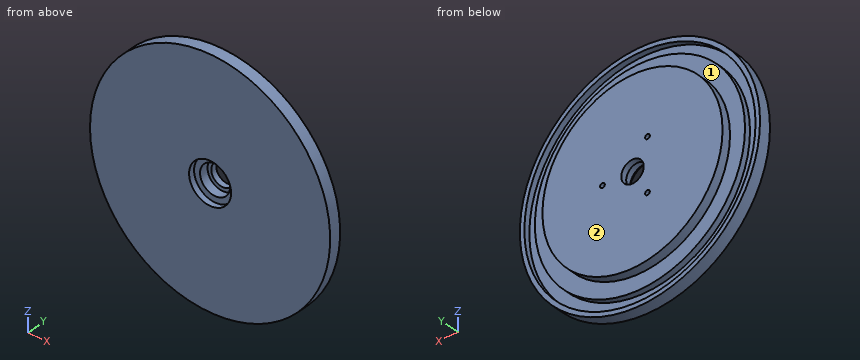
Autodesk Inventor part; units mm, degrees
ref_plane "YZ Plane" through (0, 0, 0) normal (1, 0, 0) x (0, 1, 0)
ref_plane "XZ Plane" through (0, 0, 0) normal (0, 1, 0) x (-1, 0, 0)
ref_plane "XY Plane" through (0, 0, 0) normal (0, 0, 1) x (1, 0, 0)
sketch "Sketch1" plane through (0, 0, 0) normal (0, 0, 1) x (1, 0, 0)
  line L0 (0, 0) -> (0, 5) construction
  line L1 (-40, 4) -> (-40, 0)
  line L2 (-40, 0) -> (-4.5, 0)
  line L3 (-38.5, 4) -> (-38.5, 2)
  line L4 (-38.5, 2) -> (-35, 2)
  line L5 (-35, 2) -> (-35, 4)
  line L6 (-30, 4) -> (-35, 4)
  line L7 (-38.5, 4) -> (-40, 4)
  line L8 (-3.75, 5) -> (-5, 5)
  line L9 (-5, 5) -> (-5, 2)
  line L10 (-3.5, 2.9949) -> (3.5, 2.9949)
  line L11 (3.5, 2.9949) -> (3.5, 2.0051)
  line L12 (3.5, 2.0051) -> (-3.5, 2.0051)
  line L13 (-3.5, 2.0051) -> (-3.5, 2.9949)
  line L14 (-3.5, 2.9949) -> (3.5, 2.0051) construction
  line L15 (3.5, 2.9949) -> (-3.5, 2.0051) construction
  line L16 (-30, 4) -> (-30, 7)
  line L17 (-30, 7) -> (-3.75, 7)
  line L18 (-3.75, 7) -> (-3.75, 5)
  line L19 (-5, 2) -> (-7, 2)
  line L20 (-7, 2) -> (-7, 0)
  point P0 (0, 2.5)
  dimension "d0" = 4
  dimension "d3" = 80
  dimension "d6" = 3.5
  dimension "d7" = 2
  dimension "d15" = 70
  dimension "d16" = 7
  dimension "d17" = 1.5
  dimension "d18" = 3
  dimension "d33" = 3
  dimension "d34" = 60
  dimension "d35" = 7.5
  dimension "d40" = 14
  dimension "d41" = 2
revolve "Revolution1" add sketch "Sketch1" angle 360 about axis through (0, 0, 0) along (0, 1, 0) contours L7 L3 L4 L5 L6 L16 L17 L18 L8 L9 L19 L20 L2 L1
sketch "Sketch3" plane through (0, 7, 0) normal (0, 1, 0) x (1, 0, 0)
  circle A0 centre (0, 0) radius 3.75
  point P0 (10, 0)
  dimension "d36" = 10
hole "Hole1" at (10, 7, 0) direction (0, -1, 0) diameter 1.567 depth 5 tip angle 118
pattern_circular "Circular Pattern2" count 3 over 360 about axis through (0, 5.5, 0) along (0, 1, 0) of "Hole1"
properties part number "007" material "Stainless Steel, 440C"
The listing builds one solid part. Answer for the finished solid, in the listing's coordinates (mm). Face numbers are marked on the shaded views. A direction names the side the tool comes from. Give positions to 0.01 mm unless a question says otherwise; leave off trailing zeros. Write each loop counter-clockwise with the first axis right and the second up, starting at its lowest first coordinate (ties: lowest second). Pieces come first, ordered by that corner, then holes.
Item 1: Section B-B, the plane z = -33.5 is taken. Write down the section's boundary in (x, y), plus the area to 3 significant figures.
Item 2: Section C-C, the plane x = 13 is taken. Write down the section's boundary in (y, z), plus the area to 3 significant figures.
Item 3: Section A-A, the plane x = 0 is taken. Write down the section's boundary in (y, z).
Item 4: Section D-D, the plane z = 11 is taken. Write down the section's boundary in (x, y).
Item 5: A flat-ended cylindrical pin translates along its axis: P1, Ø1.4, axis at x = -5, z = 8.66, coming from the +Y side. Find the tip coordinate at first contact, or state that the pin passes through.
Item 6: Find the intervals of material crossed by line 1 along Z through (x, y) = (0, 2.6); line 2 along Z through (x, y) = (-11.5, 3.5); line 3 along Z through (x, y) = (3, 2.5), in increasing order.
Item 7: Which of the six approach directions +Z, -Z, +X, -X, +Y, -Y give full straight-line access (tool end or side, diameter ignored) to the marked faces 1 and 2?
Completed:
1. outline: (-21.86, 0) - (21.86, 0) - (21.86, 4) - (18.97, 4) - (18.97, 2) - (10.14, 2) - (10.14, 4) - (-10.14, 4) - (-10.14, 2) - (-18.97, 2) - (-18.97, 4) - (-21.86, 4) - close
1. area: 140 mm2
2. outline: (0, -37.83) - (4, -37.83) - (4, -36.24) - (2, -36.24) - (2, -32.5) - (4, -32.5) - (4, -27.04) - (7, -27.04) - (7, 27.04) - (4, 27.04) - (4, 32.5) - (2, 32.5) - (2, 36.24) - (4, 36.24) - (4, 37.83) - (0, 37.83) - close
2. area: 450 mm2
3. outline: (0, -40) - (4, -40) - (4, -38.5) - (2, -38.5) - (2, -35) - (4, -35) - (4, -30) - (7, -30) - (7, -3.75) - (5, -3.75) - (5, -5) - (2, -5) - (2, -7) - (0, -7) - close; (0, 7) - (2, 7) - (2, 5) - (5, 5) - (5, 3.75) - (7, 3.75) - (7, 30) - (4, 30) - (4, 35) - (2, 35) - (2, 38.5) - (4, 38.5) - (4, 40) - (0, 40) - close
4. outline: (-38.46, 0) - (38.46, 0) - (38.46, 4) - (36.9, 4) - (36.9, 2) - (33.23, 2) - (33.23, 4) - (27.91, 4) - (27.91, 7) - (-27.91, 7) - (-27.91, 4) - (-33.23, 4) - (-33.23, 2) - (-36.9, 2) - (-36.9, 4) - (-38.46, 4) - close
5. P1: stops at y = 1.95
6. line 1: z = -40 to -38.5, -35 to -5, 5 to 35, 38.5 to 40
6. line 2: z = -38.31 to -36.74, -33.06 to 33.06, 36.74 to 38.31
6. line 3: z = -39.89 to -38.38, -34.87 to -4, 4 to 34.87, 38.38 to 39.89
7. face 1: +Y
7. face 2: +Z, -Z, +X, -X, +Y
